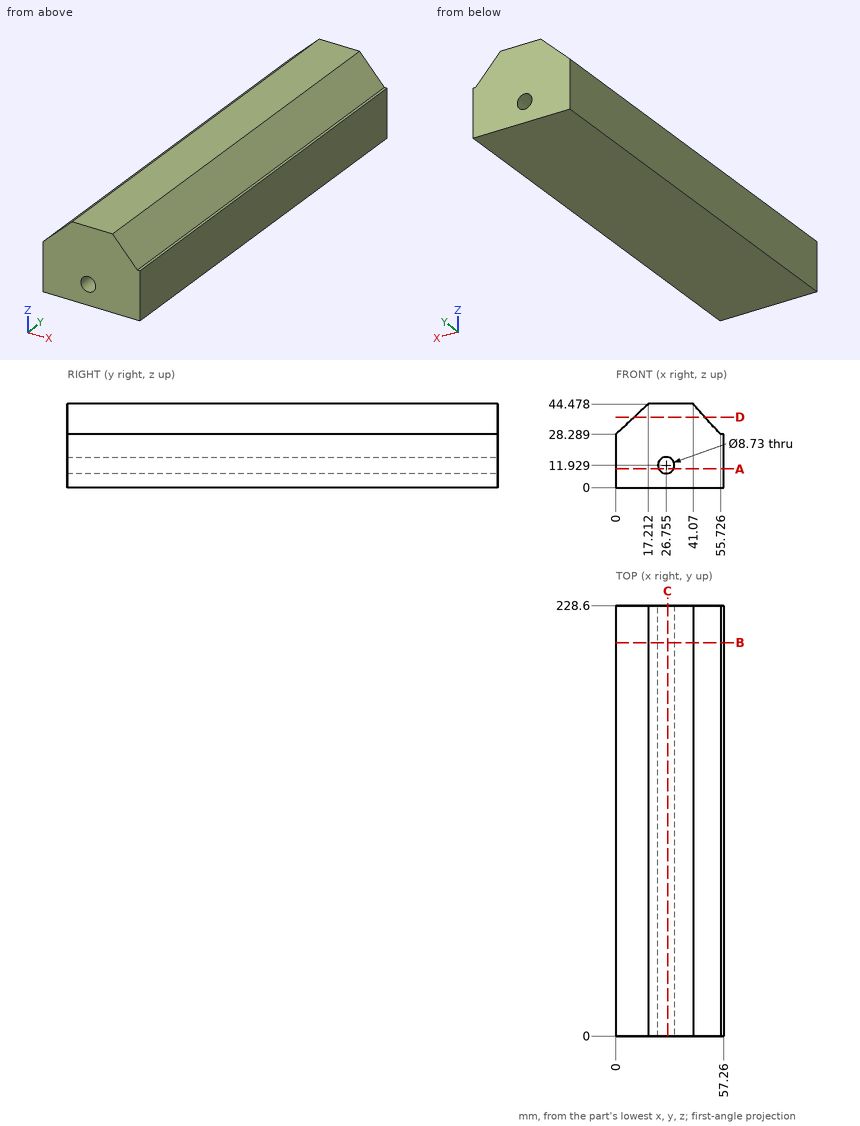
Here's the drawing with two shaded views (mm, measured from the low corner). I have some questions. Coordinates: 2 decimals unless noted, no trailing zeros. Write each loop counter-clockwise with the first axis right and the second up, starting at its lowest first coordinate (ties: lowest second). Pieces come first, ordered by that corner, then holes. Notation, with made-up numbers: M 29,-28.75 L 88,-28.75 A24 cw 88,-9.75 Z; hole C 16,67 d11. An arc over 180 degrees is marked long. Use one line per item in the form item = value.
Q1. If we section it at D-D (z = 37.5): Write out the boundary of the cut face in (x, y).
Model answer:
outline = M 9.79,0 L 47.39,0 L 47.39,228.6 L 9.79,228.6 Z
Q2. For P1, Ø0.5, axis at x = 56.5, y = 72.5, coming from the +Z side; P2, Ø2, axis at y = 61.5, z = 31, coming from the -X side; P3, Ø1, axis at y = 62, z = 33, coming from the -X side (1 decimal), each with a flat end and sliding along its axis, tell me the tip position at first contact or that it passes through.
Model answer:
P1 = 28.29
P2 = 1.82
P3 = 4.5
Q3. If we section it at B-B (y = 209): Write out the boundary of the cut face in (x, z) (1 decimal), then the cut area to 3 significant figures.
Model answer:
outline = M 0,0 L 57.3,0 L 57.3,28.3 L 55.7,28.3 L 41.1,44.5 L 17.2,44.5 L 0,28.3 Z; hole C 26.8,11.9 d8.7
area = 2,200 mm^2
Q4. If we section it at C-C (x = 27.5): Write out the boundary of the cut face in (y, z), then the cut area to 3 significant figures.
Model answer:
outline = M 0,0 L 228.6,0 L 228.6,7.63 L 0,7.63 Z; M 0,16.23 L 228.6,16.23 L 228.6,44.48 L 0,44.48 Z
area = 8,200 mm^2
Q5. I need wall thicknesses on line 1 along X through (y, z) = (62, 15) (1 decimal); line 2 along X through (y, z) = (152, 8.5) (1 decimal); line 3 along Z through (x, y) = (53, 70). Which ranges of each line are inside material? Lowest first, please. Write a range as from..to.
Model answer:
line_1 = 0..23.7, 29.9..57.3
line_2 = 0..24.1, 29.5..57.3
line_3 = 0..31.3
Q6. If we section it at A-A (z = 10): Write out the boundary of the cut face in (x, y).
Model answer:
outline = M 0,0 L 22.84,0 L 22.84,228.6 L 0,228.6 Z; M 30.67,0 L 57.26,0 L 57.26,228.6 L 30.67,228.6 Z
